from build123d import *

# Parameters (mm, degrees)
SKETCH3_W               = 12
SKETCH3_H               = 3
CHAMFER1_SIZE           = 0.75
SKETCH8_W               = 3.6
SKETCH8_H               = 6
CUT_EXTRUDE_THIN2_START = 14.3
SKETCH12_W              = 12
SKETCH12_H              = 1.9
CUT_EXTRUDE_THIN2_DEPTH = 1.3


with BuildPart() as part:
    # Sketch3 → Revolve1 (revolve)
    with BuildSketch(Plane(origin=(0, 0, 0), x_dir=(0, 0, -1), z_dir=(1, 0, 0)), mode=Mode.PRIVATE) as revolve1_sk:
        with Locations((-6, 1.5)):
            Rectangle(SKETCH3_W, SKETCH3_H)
    revolve(revolve1_sk.sketch.rotate(Axis((0, 0, 0), (0, 0, -1)), 90), axis=Axis((0, 0, 0), (0, 0, -1)))

    # Chamfer1
    chamfer1_edges = [part.edges().sort_by_distance(p)[0] for p in [
        (-3, 0, 0),
    ]]
    chamfer(chamfer1_edges, length=CHAMFER1_SIZE)

    # Sketch8 → Revolve2 (revolve)
    with BuildSketch(Plane(origin=(0, 0, 0), x_dir=(0, 0, -1), z_dir=(1, 0, 0)), mode=Mode.PRIVATE) as revolve2_sk:
        with Locations((-13.8, 3)):
            Rectangle(SKETCH8_W, SKETCH8_H)
    revolve(revolve2_sk.sketch.rotate(Axis((0, 0, 0), (0, 0, 1)), 90), axis=Axis((0, 0, 0), (0, 0, 1)))

    # Sketch11 → Cut-Revolve3 (revolve, cut)
    with BuildSketch(Plane(origin=(0, 0, 0), x_dir=(0, 0, -1), z_dir=(1, 0, 0)), mode=Mode.PRIVATE) as cut_revolve3_sk:
        with BuildLine():
            Line((-14.34, 6), (-12.54, 6))
            ThreePointArc((-12.54, 6), (-12.158162338, 5.841837662), (-12, 5.46))
            Line((-12, 5.46), (-11.365, 5.46))
            Line((-11.365, 5.46), (-11.365, 6.635))
            Line((-11.365, 6.635), (-16.235, 6.635))
            Line((-16.235, 6.635), (-16.235, 0))
            Line((-16.235, 0), (-15.6, 0))
            ThreePointArc((-15.6, 0), (-15.41458949, 2.824231581), (-14.861540653, 5.599983383))
            ThreePointArc((-14.861540653, 5.599983383), (-14.668640361, 5.88848047), (-14.34, 6))
        make_face()
    revolve(cut_revolve3_sk.sketch.rotate(Axis((0, 0, 15.6), (0, 0, -1)), 180), axis=Axis((0, 0, 15.6), (0, 0, -1)), mode=Mode.SUBTRACT)

    # Sketch12 → Cut-Extrude-Thin2 (cut)
    with BuildSketch(Plane.XY.offset(CUT_EXTRUDE_THIN2_START)):
        Rectangle(SKETCH12_W, SKETCH12_H)
    extrude(amount=CUT_EXTRUDE_THIN2_DEPTH, mode=Mode.SUBTRACT)


solid = part.part
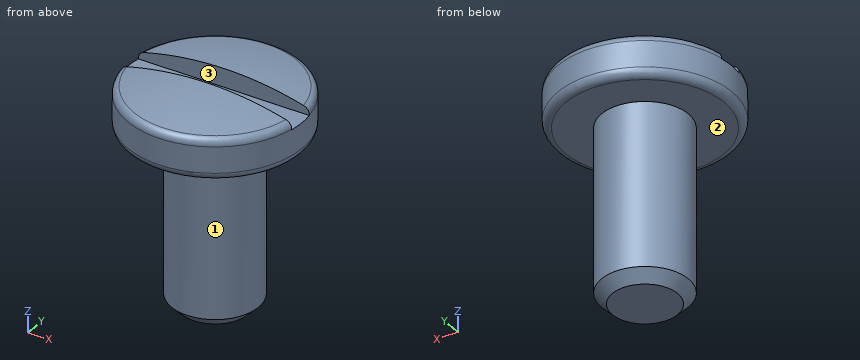
The model under review builds one solid part; all positions refer to its coordinate system, in mm. Face numbers are marked on the shaded views. Round coordinates to 2 decimals unless told otherwise and drop trailing zeros. Write each loop counter-clockwise with the first axis right and the second up, starting at its lowest first coordinate (ties: lowest second). Pieces come first, ordered by that corner, then holes. Notation, with made-up numbers: (16, 59.5) -> (57, 59.5) arc R16 cw to (57, 81.5) -> close; hole circle Ø8 at (84, -18.75). An arc over 180 degrees is marked (long way). Answer as a JSON object with one key per item and string values.
1. Clearance check with flat-ended pins moving along their axes: pin 1 (5 mm diameter, centred on x = 3.5, y = -4, fed in from -Z); pin 2 (4 mm diameter, centred on y = 4.5, z = 4, fed in from +X); pin 3 (5.5 mm diameter, centred on x = -0.5, y = 0, fed in from -Z); pin 4 (5 mm diameter, centred on x = -3.5, z = 10.5, fed in from -Y). State where each tip first meets the part, or that it passes through.
Results found:
{"pin 1": "stops at z = 0.57", "pin 2": "stops at x = 1.66", "pin 3": "stops at z = 0", "pin 4": "stops at y = -5.68"}
2. We need section B-B on z = 9.5. State the section outline as (x, y) points.
Results found:
{"outline": "circle Ø6 at (0, 0)"}
3. The part is to be moulded in two halves that separate along Y. For the marked faces 1, 2 and 3, say which applies: pulls with the +Y half, pulls with the -Y half, needs draft (parallel to the pull), parting line crosses it, or undercut.
Results found:
{"face 1": "parting line crosses it", "face 2": "needs draft", "face 3": "undercut"}
4. To check wall thickness, follow line 1 along X through (y, z) = (-1.25, 4); line 2 along Z through (x, y) = (2.25, -1.25); line 3 along Y through (x, z) = (0.75, 13). State the ranges of each line that lie inside material, in increasing order.
Results found:
{"line 1": "x = -2.73 to 2.73", "line 2": "z = 0.32 to 15.45", "line 3": "y = -5.95 to 5.95"}
